The drawing under review shows one solid part. Ordinate dimensions are in mm from its lowest x, y, z. A direction names the side the tool comes from. Give positions to 0.01 mm unless a question says otherwise; leave off trailing zeros. Loops run counter-clockwise (first coordinate to the right, second up) from the corner with the lowest first, then second, coordinate; pieces in that order, holes last. Notation, with made-up numbers: (39.25, 22) - (68.25, 22) arc R7 cw to (68.25, 31) - close; hole circle Ø6 at (89, 61). An arc over 180 degrees is marked (long way). Answer as CSV lines item,"result".
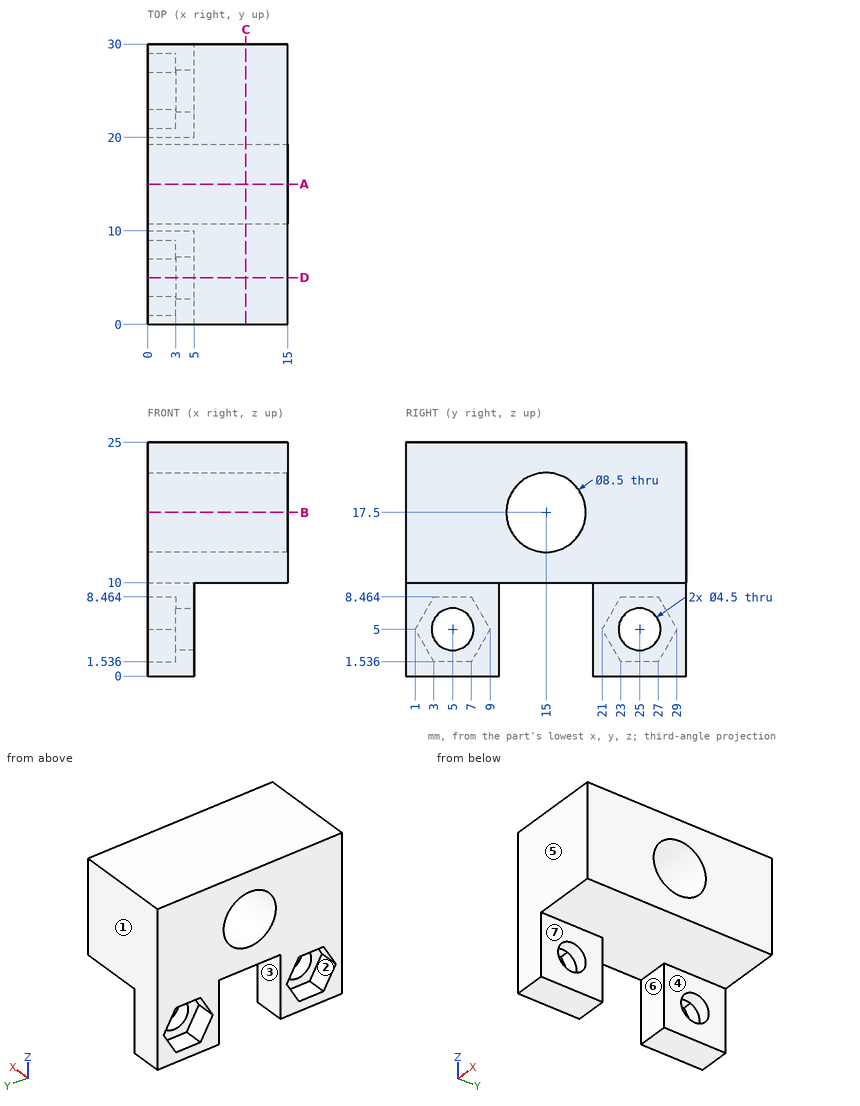
1) Draft analysis for pull direction Y (two halves, no side actions). For the marked faces 5, 6 and 7, state which applies: pulls with the +Y half, pulls with the -Y half, needs draft (parallel to the pull), parting line crosses it, or undercut.
From the geometry:
face 5,"pulls with the -Y half"
face 6,"undercut"
face 7,"needs draft"
2) Consider section B-B on z = 17.5. Write out the cut boundary in (x, y), and give its area (4 significant figures).
From the geometry:
outline,"(0, 0) - (15, 0) - (15, 10.75) - (0, 10.75) - close; (0, 19.25) - (15, 19.25) - (15, 30) - (0, 30) - close"
area,"322.5 mm^2"
3) Wall thickness on line 1 (Y direction, x = 3.5, z = 5); line 2 (Y direction, x = 9, z = 17.5); line 3 (Z direction, x = 10, y = 8): over which ranges is each line inside the solid? List them lowest first. Write a range as from..to.
From the geometry:
line 1,"y = 0..2.75, 7.25..10, 20..22.75, 27.25..30"
line 2,"y = 0..10.75, 19.25..30"
line 3,"z = 10..25"
4) Insertion check: P1, Ø5, axis at y = 5, z = 5, coming from the +X side; P2, Ø5.5, axis at y = 25, z = 5, coming from the -X side. Each pin has a flat end and moves straight along its axis. Give the tip position at first contact, or say it passes through.
From the geometry:
P1,"stops at x = 5"
P2,"stops at x = 3"
5) Consider section D-D on y = 5. Write out the cut boundary in (x, z), and give its area (3 significant figures).
From the geometry:
outline,"(0, 0) - (5, 0) - (5, 2.75) - (3, 2.75) - (3, 1.54) - (0, 1.54) - close; (0, 8.46) - (3, 8.46) - (3, 7.25) - (5, 7.25) - (5, 10) - (15, 10) - (15, 25) - (0, 25) - close"
area,"245 mm^2"
6) Consider section A-A on y = 15. Write out the cut boundary in (x, z).
From the geometry:
outline,"(0, 10) - (15, 10) - (15, 13.25) - (0, 13.25) - close; (0, 21.75) - (15, 21.75) - (15, 25) - (0, 25) - close"
7) Machinability: for the marked faces 1, 2, 3 and 4, which of the approach directions +Z, -Z, +X, -X, +Y, -Y give a long, thin tool a straight path to every point of the face, cutting with its end or side? Answer none if there is none.
From the geometry:
face 1,"+Z, -Z, +X, -X, +Y"
face 2,"-X"
face 3,"-Z, +X, -X"
face 4,"-Z, +X, +Y, -Y"
8) Consider section C-C on x = 10.5. Write out the cut boundary in (y, z).
From the geometry:
outline,"(0, 10) - (30, 10) - (30, 25) - (0, 25) - close; hole circle Ø8.5 at (15, 17.5)"
